Source: CAD feature listing. Evaluate the final solid. Frame: model axes, mm. Face numbers are marked on the shaded views. A direction names the side the tool comes from. Round coordinates to 2 decimals unless told otherwise and drop trailing zeros. Order: outer loops, then holes, each group sorted by start corner. A loop starts at its lowest first (then second) coordinate and runs counter-clockwise, first axis right, second up. Notation, with made-up numbers: M 49.5,61 L 85.5,61 A20 cw 85.5,97 Z; hole C 10,7 d4. An arc over 180 degrees is marked long. Use one line per item in the form item = value. Start each with the question number.
Q1. Pull-direction query (Z, two-part tool) for the marked faces 1, 2 and 3; classes: pulls with the +Z half, pulls with the -Z half, needs draft (parallel to the pull), parting line crosses it, or undercut.
Q2. Section B-B (x = 0). Return the cut outline in (y, z), plus the area to 3 significant figures.
Q3. Contact query for flat-ended pins moving along their axis: pin 1 (8 mm diameter, centred on x = 0.5, z = 4, fed in from +Y); pin 2 (2 mm diameter, centred on y = -9.5, z = -4.5, fed in from -X); pin 3 (6 mm diameter, centred on x = -7, y = -5, fed in from -Z); pin 4 (5 mm diameter, centred on x = 2.5, z = -10, fed in from +Y). Output: stop coordinate, or through.
Q4. Material intervals for probe 1 along Z at (x, y) = (0, -9); probe 2 along Z at (x, y) = (0, -11.7); probe 3 along Y at (x, z) = (-1.5, -5.25), sorted ascending.
Q5. Section C-C (z = 8.5). Return the cut outline in (x, y).
Q6. Reachability of the marked faces 4, 5 and 6 from +Z, -Z, +X, -X, +Y, -Y: full face, straight path, thin tool, end or side. Return the list, or none.
Q7. Section A-A (y = -3.5). Return the cut outline in (x, z), plus the area to 3 significant figures.
Q8. Section D-D (y = -2). Return the cut outline in (x, z).
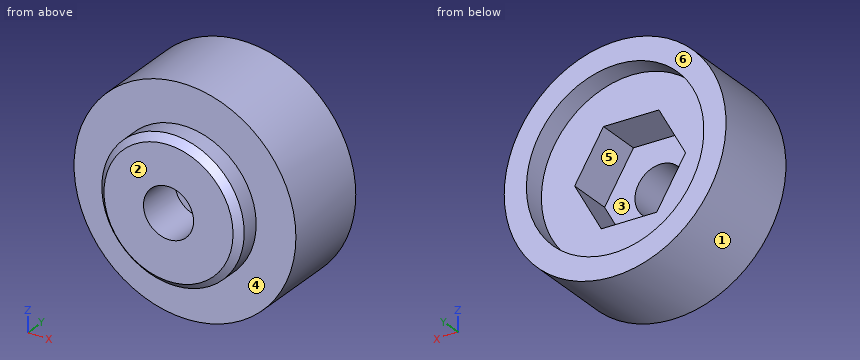
from build123d import *

# Parameters (mm, degrees)
F0_R     = 12.7
F0_R_2   = 10.16
F0_R_3   = 8.1534
F0_R_4   = 2.8702
F1_DEPTH = 10.16
F2_DEPTH = 12.954
F3_DEPTH = 2.54
F4_DEPTH = 7.62
F5_SIZE  = 0.762


with BuildPart() as f1:
    # F0 (on Front) → F1 (new body)
    with BuildSketch(Plane.XZ):
        Circle(F0_R)
        Circle(F0_R_2, mode=Mode.SUBTRACT)
        Circle(F0_R_2)
        Circle(F0_R_3, mode=Mode.SUBTRACT)
        Circle(F0_R_3)
        Polygon((-3.299791, 5.425082), (3.048363, 5.570244), (6.348154, 0.145162), (3.299791, -5.425082), (-3.048363, -5.570244), (-6.348154, -0.145162), align=None, mode=Mode.SUBTRACT)
        Polygon((6.348154, 0.145162), (3.048363, 5.570244), (-3.299791, 5.425082), (-6.348154, -0.145162), (-3.048363, -5.570244), (3.299791, -5.425082), align=None)
        Circle(F0_R_4, mode=Mode.SUBTRACT)
    extrude(amount=F1_DEPTH)

    # F0 (on Front) → F2 (join)
    with BuildSketch(Plane.XZ):
        Circle(F0_R_3)
        Polygon((-3.299791, 5.425082), (3.048363, 5.570244), (6.348154, 0.145162), (3.299791, -5.425082), (-3.048363, -5.570244), (-6.348154, -0.145162), align=None, mode=Mode.SUBTRACT)
        Polygon((6.348154, 0.145162), (3.048363, 5.570244), (-3.299791, 5.425082), (-6.348154, -0.145162), (-3.048363, -5.570244), (3.299791, -5.425082), align=None)
        Circle(F0_R_4, mode=Mode.SUBTRACT)
    extrude(amount=F2_DEPTH)

    # F0 (on Front) → F3 (cut)
    with BuildSketch(Plane.XZ):
        Circle(F0_R_2)
        Circle(F0_R_3, mode=Mode.SUBTRACT)
        Circle(F0_R_3)
        Polygon((-3.299791, 5.425082), (3.048363, 5.570244), (6.348154, 0.145162), (3.299791, -5.425082), (-3.048363, -5.570244), (-6.348154, -0.145162), align=None, mode=Mode.SUBTRACT)
        Polygon((6.348154, 0.145162), (3.048363, 5.570244), (-3.299791, 5.425082), (-6.348154, -0.145162), (-3.048363, -5.570244), (3.299791, -5.425082), align=None)
        Circle(F0_R_4, mode=Mode.SUBTRACT)
    extrude(amount=F3_DEPTH, mode=Mode.SUBTRACT)

    # F0 (on Front) → F4 (cut)
    with BuildSketch(Plane.XZ):
        Polygon((6.348154, 0.145162), (3.048363, 5.570244), (-3.299791, 5.425082), (-6.348154, -0.145162), (-3.048363, -5.570244), (3.299791, -5.425082), align=None)
        Circle(F0_R_4, mode=Mode.SUBTRACT)
    extrude(amount=F4_DEPTH, mode=Mode.SUBTRACT)

    # F5
    f5_edges = [f1.edges().sort_by_distance(p)[0] for p in [
        (-8.1534, -12.954, 0),
    ]]
    chamfer(f5_edges, length=F5_SIZE)


solid = f1.part
Results list:
q1.face_1 = parting line crosses it
q1.face_2 = needs draft
q1.face_3 = undercut
q2.outline = M -12.95,-7.39 L -12.19,-8.15 L -10.16,-8.15 L -10.16,-12.7 L 0,-12.7 L 0,-10.16 L -2.54,-10.16 L -2.54,-5.5 L -7.62,-5.5 L -7.62,-2.87 L -12.95,-2.87 Z; M -12.95,2.87 L -7.62,2.87 L -7.62,5.5 L -2.54,5.5 L -2.54,10.16 L 0,10.16 L 0,12.7 L -10.16,12.7 L -10.16,8.15 L -12.19,8.15 L -12.95,7.39 Z
q2.area = 165 mm2
q3.pin_1 = -2.54
q3.pin_2 = -12.21
q3.pin_3 = -12.05
q3.pin_4 = 0
q4.probe_1 = -12.7 to -2.87, 2.87 to 12.7
q4.probe_2 = -8.15 to -2.87, 2.87 to 8.15
q4.probe_3 = -12.95 to -7.62
q5.outline = M -9.44,-10.16 L 9.44,-10.16 L 9.44,0 L 5.57,0 L 5.57,-2.54 L -5.57,-2.54 L -5.57,0 L -9.44,0 Z
q6.face_4 = -Y
q6.face_5 = +Y
q6.face_6 = +Z, -Z, +X, -X, +Y
q7.outline = C 0,0 d25.4; hole M -6.35,-0.15 L -3.05,-5.57 L 3.3,-5.43 L 6.35,0.15 L 3.05,5.57 L -3.3,5.43 Z
q7.area = 402 mm2
q8.outline = C 0,0 d25.4; hole C 0,0 d20.32
